Design review of the part built by this model. Coordinates are the model's own, in mm. A direction names the side the tool comes from. Round coordinates to 2 decimals unless told otherwise and drop trailing zeros. Loops run counter-clockwise (first coordinate to the right, second up) from the corner with the lowest first, then second, coordinate; pieces in that order, holes last. Notation, with made-up numbers: (77.25, 0) - (130.25, 0) arc R18 cw to (130.25, 5) - close; hole circle Ø11 at (14.5, 65.25). An arc over 180 degrees is marked (long way). Answer as CSV lines item,"result". Start each with the question number.
(1) For P1, Ø5, axis at y = 18, z = 0, coming from the +X side; P2, Ø3, axis at x = 6, z = 0, coming from the -Y side; P3, Ø5.5, axis at y = 17, z = -2, coming from the -X side, all flat-tipped, find the tip position at first contact; note any pin that passes through.
(2) For faces 1 (the cylindrical face through (7.385, 3.549, -2.417)), 2 (the flat face through (11, 20.6, -4.5)), 3 (the flat face through (2, 29, 8)), list the 3-axis set-ups (+Z, -Z, +X, -X, +Y, -Y) from which the entire face can be reached by the end or side of a thin tool; tool diameter is ignored.
(3) Consider section A-A (x = -3.5). Give the boundary of the cut face in (y, z).
(4) Consider section C-C (z = 2). Count the separate pieces of the cut face and the enclosed holes in it, and give its area (3 significant figures).
(5) Consider section B-B (x = 11). Give the boundary of the cut face in (y, z), and give its area (3 significant figures).
(6) Mouldability with a two-part tool opening along Y and no side actions: class faces 4 (the flat face through (9, 0, 0)), 5 (the flat face through (21.5, 18, 4)), 6 (the flat face through (-13.4, 12.5, -0.2)), 7 (the flat face through (11, 15.4, 4.5)) as released by +Y, released by -Y, zero draft, split by the parting line, or undercut.
(7) Wall thickness on L1, parallel to Z at x = -3, y = 3; L2, parallel to X at y = 26.8, z = 0; L3, parallel to Y at x = 4, z = -11: over which ranges is each line inside the solid? List them lowest first.
(8) Consider section D-D (y = 16.5). Give the boundary of the cut face in (x, z), and give its area (3 significant figures).
from build123d import *

# Parameters (mm, degrees)
SKETCH1_W           = 43
SKETCH1_H           = 30
BOSS_EXTRUDE1_DEPTH = 36
SKETCH2_W           = 30
SKETCH2_H           = 11
CUT_EXTRUDE1_DEPTH  = 30
SKETCH3_R           = 11.15
CUT_EXTRUDE2_DEPTH  = 7
CUT_EXTRUDE3_START  = -7
SKETCH4_R           = 11.15
CUT_EXTRUDE3_DEPTH  = 7
SKETCH5_R           = 9.5
CUT_EXTRUDE4_DEPTH  = 40.092838219
CUT_EXTRUDE5_DEPTH  = 5
SKETCH7_R           = 3
CUT_EXTRUDE6_DEPTH  = 53.402290026
FILLET2_R           = 15


with BuildPart() as part:
    # Sketch1 → Boss-Extrude1 (new body)
    with BuildSketch(Plane(origin=(0, 0, 0), x_dir=(1, 0, 0), z_dir=(0, 1, 0))):
        Rectangle(SKETCH1_W, SKETCH1_H)
    extrude(amount=BOSS_EXTRUDE1_DEPTH)

    # Sketch2 → Cut-Extrude1 (cut)
    with BuildSketch(Plane.ZY.offset(21.5)):
        with Locations((0, 18)):
            Rectangle(SKETCH2_W, SKETCH2_H)
    extrude(amount=-CUT_EXTRUDE1_DEPTH, mode=Mode.SUBTRACT)

    # Sketch3 → Cut-Extrude2 (cut)
    with BuildSketch(Plane(origin=(0, 36, 0), x_dir=(1, 0, 0), z_dir=(0, 1, 0))):
        with Locations(Location((-3.5, 0, 0), (0, 0, 270))):
            Circle(SKETCH3_R)
    extrude(amount=-CUT_EXTRUDE2_DEPTH, mode=Mode.SUBTRACT)

    # Sketch4 → Cut-Extrude3 (cut)
    with BuildSketch(Plane.XZ.offset(CUT_EXTRUDE3_START)):
        with Locations(Location((-3.5, 0, 0), (0, 0, 90))):
            Circle(SKETCH4_R)
    extrude(amount=CUT_EXTRUDE3_DEPTH, mode=Mode.SUBTRACT)

    # Sketch5 → Cut-Extrude4 (cut, through all)
    with BuildSketch(Plane(origin=(0, 29, 0), x_dir=(1, 0, 0), z_dir=(0, 1, 0))):
        with Locations(Location((-3.5, 0, 0), (0, 0, 90))):
            Circle(SKETCH5_R)
    extrude(amount=-CUT_EXTRUDE4_DEPTH, mode=Mode.SUBTRACT)

    # Sketch6 → Cut-Extrude5 (cut)
    with BuildSketch(Plane.ZY.offset(-8.5)):
        Polygon((-3, 23.196152423), (-6, 18), (-3, 12.803847577), (3, 12.803847577), (6, 18), (3, 23.196152423), align=None)
    extrude(amount=-CUT_EXTRUDE5_DEPTH, mode=Mode.SUBTRACT)

    # Sketch7 → Cut-Extrude6 (cut, through all)
    with BuildSketch(Plane.ZY.offset(-13.5)):
        with Locations((0, 18)):
            Circle(SKETCH7_R)
    extrude(amount=-CUT_EXTRUDE6_DEPTH, mode=Mode.SUBTRACT)

    # Fillet2
    fillet2_edges = [part.edges().sort_by_distance(p)[0] for p in [
        (-21.5, 6.25, -15),
        (-21.5, 6.25, 15),
        (-21.5, 29.75, 15),
        (-21.5, 29.75, -15),
    ]]
    fillet(fillet2_edges, radius=FILLET2_R - 0.0001)  # a hair under: the kernel refuses the full size


solid = part.part
Determined:
1,P1,"passes through"
1,P2,"stops at y = 7"
1,P3,"stops at x = 13.5"
2,face 1,"-Y"
2,face 2,"-X"
2,face 3,"+Y"
3,outline,"(0, -15) - (12.5, -15) - (12.5, -9.5) - (7, -9.5) - (7, -11.15) - (0, -11.15) - close; (0, 11.15) - (7, 11.15) - (7, 9.5) - (12.5, 9.5) - (12.5, 15) - (0, 15) - close; (23.5, -15) - (36, -15) - (36, -11.15) - (29, -11.15) - (29, -9.5) - (23.5, -9.5) - close; (23.5, 9.5) - (29, 9.5) - (29, 11.15) - (36, 11.15) - (36, 15) - (23.5, 15) - close"
4,separate pieces,"4"
4,enclosed holes,"0"
4,area,"615 mm^2"
5,outline,"(0, -15) - (36, -15) - (36, 15) - (0, 15) - close; hole (12.8, -3) - (18, -6) - (23.2, -3) - (23.2, 3) - (18, 6) - (12.8, 3) - close"
5,area,"986 mm^2"
6,face 4,"released by -Y"
6,face 5,"zero draft"
6,face 6,"undercut"
6,face 7,"undercut"
7,L1,"z = -15 to -11.14, 11.14 to 15"
7,L2,"x = -21.5 to -13, 6 to 21.5"
7,L3,"y = 0 to 12.5, 23.5 to 36"
8,outline,"(8.5, -15) - (21.5, -15) - (21.5, -2.6) - (13.5, -2.6) - (13.5, -5.13) - (8.5, -5.13) - close; (8.5, 5.13) - (13.5, 5.13) - (13.5, 2.6) - (21.5, 2.6) - (21.5, 15) - (8.5, 15) - close"
8,area,"297 mm^2"
